from build123d import *

# Parameters (mm, degrees)
F2_R     = 7.5
F3_DEPTH = 5
F4_R     = 55
F4_R_2   = 28
F5_DEPTH = 2.5
F6_R     = 1


with BuildPart() as f1:
    # F0 (on Top) → F1 (revolve)
    with BuildSketch(Plane.XY):
        Polygon((-37, 27), (0, 27), (0, 50), (-2.5, 50), (-2.5, 30), (-34.5, 30), (-34.5, 50), (-37, 50), align=None)
    revolve(axis=Axis((5.071359, 0, 0), (1, 0, 0)))

    # F2 (on face) → F3 (cut)
    with BuildSketch(Plane(origin=(-37, 0, 0), x_dir=(0, -1, 0), z_dir=(-1, 0, 0))):
        with Locations((0, 39.5)):
            Circle(F2_R)
        with Locations((-27.930718, 27.930718)):
            Circle(F2_R)
        with Locations((-39.5, 0)):
            Circle(F2_R)
        with Locations((-27.930718, -27.930718)):
            Circle(F2_R)
        with Locations((0, -39.5)):
            Circle(F2_R)
        with Locations((27.930718, -27.930718)):
            Circle(F2_R)
        with Locations((39.5, 0)):
            Circle(F2_R)
        with Locations((27.930718, 27.930718)):
            Circle(F2_R)
    extrude(amount=-F3_DEPTH, mode=Mode.SUBTRACT)

    # F4 (on face) → F5 (cut)
    with BuildSketch(Plane.YZ):
        Circle(F4_R)
        Circle(F4_R_2, mode=Mode.SUBTRACT)
    extrude(amount=-F5_DEPTH, mode=Mode.SUBTRACT)

    # F6
    f6_edges = [f1.edges().sort_by_distance(p)[0] for p in [
        (-34.5, -30, 0),
    ]]
    fillet(f6_edges, radius=F6_R)


solid = f1.part
Design review of the part built by this model. Coordinates are the model's own, in mm. A direction names the side the tool comes from. Coordinates: 2 decimals unless noted, no trailing zeros. Loops run counter-clockwise (first coordinate to the right, second up) from the corner with the lowest first, then second, coordinate; pieces in that order, holes last. Notation, with made-up numbers: (27, -24) - (75, -24) arc R17 ccw to (75, 3) - close; hole circle Ø10 at (-5, -4). An arc over 180 degrees is marked (long way). Use CSV: the item, a comma, the result in double quotes. Start each with the question number.
1. Add section D-D on x = -18.5. Give the boundary of the cut face in (y, z).
2. Add section C-C on y = 0. Give the boundary of the cut face in (x, z).
3. For faces 4 (the cylindrical face through (-18.22, -29.97, 1.32)), 5 (the cylindrical face through (-35.768, -22.403, -22.862)), list the 3-axis set-ups (+Z, -Z, +X, -X, +Y, -Y) from which the entire face can be reached by the end or side of a thin tool; tool diameter is ignored.
4. Mouldability with a two-part tool opening along Z and no side actions: class faces 1 (the flat face through (-37, 22, -22)), 2 (the cylindrical face through (-35.77, 47.69, 15.02)), 3 (the cylindrical face through (-35.77, 29.56, 20.61)) as released by +Z, released by -Z, zero draft, split by the parting line, or undercut.
5. To check wall thickness, follow probe 1 along Z at (x, y) = (-36.5, 0); probe 2 along X at (y, z) = (-19.5, 28); probe 3 along Y at (x, z) = (-1.5, 10). State the ranges of each line that lie inside material, in increasing order.
6. Clearance check with flat-ended pins moving along their axes: pin 1 (1 mm diameter, centred on x = -22.5, y = 24, fed in from +Z); pin 2 (4 mm diameter, centred on x = -23.5, z = 18, fed in from +Y); pin 3 (10 mm diameter, centred on x = -25.5, z = -30, fed in from -Y). State where each tip first meets the part, or that it passes through.
7. Add section A-A on z = 39.5. Give the boundary of the cut face in (x, y).
Resolved:
1,outline,"circle Ø60 at (0, 0); hole circle Ø54 at (0, 0)"
2,outline,"(-37, -50) - (-34.5, -50) - (-34.5, -47) - (-37, -47) - close; (-37, -32) - (-34.5, -32) - (-34.5, -31) arc R1 cw to (-33.5, -30) - (-2.5, -30) - (-2.5, -28) - (0, -28) - (0, -27) - (-37, -27) - close; (-37, 27) - (0, 27) - (0, 28) - (-2.5, 28) - (-2.5, 30) - (-33.5, 30) arc R1 cw to (-34.5, 31) - (-34.5, 32) - (-37, 32) - close; (-37, 47) - (-34.5, 47) - (-34.5, 50) - (-37, 50) - close"
3,face 4,"+X"
3,face 5,"+X, -X"
4,face 1,"zero draft"
4,face 2,"split by the parting line"
4,face 3,"undercut"
5,probe 1,"-50 to -47, -32 to -27, 27 to 32, 47 to 50"
5,probe 2,"-37 to -34.5"
5,probe 3,"-26.15 to -25.08, 25.08 to 26.15"
6,pin 1,"z = 18.65"
6,pin 2,"y = 25.38"
6,pin 3,"y = -16.58"
7,outline,"(-37, -30.66) - (-34.5, -30.66) - (-34.5, -7.5) - (-37, -7.5) - close; (-37, 7.5) - (-34.5, 7.5) - (-34.5, 30.66) - (-37, 30.66) - close"
